from build123d import *

# Parameters (mm, degrees)
CROQUIS1_W                       = 60
CROQUIS1_H                       = 60
SALIENTE_EXTRUIR1_DEPTH          = 73
CORTAR_EXTRUIR1_REACH            = 101.141
CROQUIS2_W                       = 50
CROQUIS2_H                       = 69.5
CORTAR_EXTRUIR2_REACH            = 86.433
CROQUIS3_R                       = 2
CHAFL_N1_SIZE                    = 5
TALADRO_DE_MARGEN_PARA_M31_D     = 3.4
TALADRO_DE_MARGEN_PARA_M31_DEPTH = 40
TALADRO_DE_MARGEN_PARA_M31_TIP   = 1.021463052
TALADRO_DE_MARGEN_PARA_M32_D     = 3.4
TALADRO_DE_MARGEN_PARA_M32_DEPTH = 40
TALADRO_DE_MARGEN_PARA_M32_TIP   = 1.021463052
TALADRO_DE_MARGEN_PARA_M33_D     = 3.4
TALADRO_DE_MARGEN_PARA_M33_DEPTH = 40
TALADRO_DE_MARGEN_PARA_M33_TIP   = 1.021463052
CROQUIS11_W                      = 60
CROQUIS11_H                      = 3.5
SALIENTE_EXTRUIR2_DEPTH          = 40
CHAFL_N2_SIZE                    = 40
CORTAR_EXTRUIR3_REACH            = 107.494
CROQUIS12_R                      = 2.5
CROQUIS14_R                      = 10
SALIENTE_EXTRUIR3_DEPTH          = 7
CROQUIS15_R                      = 10
SALIENTE_EXTRUIR4_DEPTH          = 2
CROQUIS13_R                      = 8
CORTAR_EXTRUIR5_DEPTH            = 5
CROQUIS16_R                      = 5
CORTAR_EXTRUIR6_DEPTH            = 5
CROQUIS17_R                      = 4.5
CORTAR_EXTRUIR7_DEPTH            = 16


with BuildPart() as part:
    # Croquis1 → Saliente-Extruir1 (new body)
    with BuildSketch(Plane(origin=(0, 0, 0), x_dir=(1, 0, 0), z_dir=(0, 1, 0))):
        Rectangle(CROQUIS1_W, CROQUIS1_H)
    extrude(amount=SALIENTE_EXTRUIR1_DEPTH)

    # Croquis2 → Cortar-Extruir1 (cut, up to next)
    with BuildSketch(Plane.XY.offset(30), mode=Mode.PRIVATE) as cortar_extruir1_sk1:
        with Locations((0, 34.75)):
            Rectangle(CROQUIS2_W, CROQUIS2_H)
    cortar_extruir1_tool1 = extrude(cortar_extruir1_sk1.sketch, amount=-CORTAR_EXTRUIR1_REACH, mode=Mode.PRIVATE) & part.part
    add(cortar_extruir1_tool1.solids().sort_by_distance((0, 34.75, 30))[0], mode=Mode.SUBTRACT)

    # Croquis3 → Cortar-Extruir2 (cut, up to next)
    with BuildSketch(Plane(origin=(0, 73, 0), x_dir=(1, 0, 0), z_dir=(0, 1, 0)), mode=Mode.PRIVATE) as cortar_extruir2_sk1:
        with Locations(Location((-8.5, -5.5, 0), (0, 0, 270))):
            Circle(CROQUIS3_R)
    cortar_extruir2_tool1 = extrude(cortar_extruir2_sk1.sketch, amount=-CORTAR_EXTRUIR2_REACH, mode=Mode.PRIVATE) & part.part
    # Croquis3 → Cortar-Extruir2 (cut, up to next)
    with BuildSketch(Plane(origin=(0, 73, 0), x_dir=(1, 0, 0), z_dir=(0, 1, 0)), mode=Mode.PRIVATE) as cortar_extruir2_sk2:
        with Locations(Location((8.5, -5.5, 0), (0, 0, 270))):
            Circle(CROQUIS3_R)
    cortar_extruir2_tool2 = extrude(cortar_extruir2_sk2.sketch, amount=-CORTAR_EXTRUIR2_REACH, mode=Mode.PRIVATE) & part.part
    add(cortar_extruir2_tool1.solids().sort_by_distance((-8.5, 73, 5.5))[0], mode=Mode.SUBTRACT)
    add(cortar_extruir2_tool2.solids().sort_by_distance((8.5, 73, 5.5))[0], mode=Mode.SUBTRACT)

    # Chaflán1
    chafl_n1_edges = [part.edges().sort_by_distance(p)[0] for p in [
        (-25, 69.5, 0),
        (25, 69.5, 0),
    ]]
    chamfer(chafl_n1_edges, length=CHAFL_N1_SIZE)

    # Taladro de margen para M31
    with Locations(Plane.XZ):
        with Locations((27.5, -20), (27.5, 20)):
            Hole(TALADRO_DE_MARGEN_PARA_M31_D / 2, depth=TALADRO_DE_MARGEN_PARA_M31_DEPTH)
            with Locations((0, 0, -(TALADRO_DE_MARGEN_PARA_M31_DEPTH + TALADRO_DE_MARGEN_PARA_M31_TIP / 2))):  # 118° drill point
                Cone(0, TALADRO_DE_MARGEN_PARA_M31_D / 2, TALADRO_DE_MARGEN_PARA_M31_TIP, mode=Mode.SUBTRACT)

    # Taladro de margen para M32
    with Locations(Plane.XZ):
        with Locations((-27.5, 20), (-27.5, -20)):
            Hole(TALADRO_DE_MARGEN_PARA_M32_D / 2, depth=TALADRO_DE_MARGEN_PARA_M32_DEPTH)
            with Locations((0, 0, -(TALADRO_DE_MARGEN_PARA_M32_DEPTH + TALADRO_DE_MARGEN_PARA_M32_TIP / 2))):  # 118° drill point
                Cone(0, TALADRO_DE_MARGEN_PARA_M32_D / 2, TALADRO_DE_MARGEN_PARA_M32_TIP, mode=Mode.SUBTRACT)

    # Taladro de margen para M33
    with Locations(Plane.XZ):
        with Locations((-27.5, 0), (27.5, 1.783505525)):
            Hole(TALADRO_DE_MARGEN_PARA_M33_D / 2, depth=TALADRO_DE_MARGEN_PARA_M33_DEPTH)
            with Locations((0, 0, -(TALADRO_DE_MARGEN_PARA_M33_DEPTH + TALADRO_DE_MARGEN_PARA_M33_TIP / 2))):  # 118° drill point
                Cone(0, TALADRO_DE_MARGEN_PARA_M33_D / 2, TALADRO_DE_MARGEN_PARA_M33_TIP, mode=Mode.SUBTRACT)

    # Croquis11 → Saliente-Extruir2 (add)
    with BuildSketch(Plane.XY.offset(30)):
        with Locations((0, 71.25)):
            Rectangle(CROQUIS11_W, CROQUIS11_H)
    extrude(amount=SALIENTE_EXTRUIR2_DEPTH)

    # Chaflán2
    # the kernel refuses this chamfer: 40 mm, written as the material it adds along each edge
    with BuildSketch(Plane(origin=(30, 69.5, 30), x_dir=(0, -0.9996219169112968, -0.027495876610586403), z_dir=(-1, 0, 0))) as chafl_n2_piece_1_section:
        Polygon((CHAFL_N2_SIZE * 0.999621916911, CHAFL_N2_SIZE * 0.0274958766106), (-CHAFL_N2_SIZE * 0.0274958766106, CHAFL_N2_SIZE * 0.999621916911), (0, 0), align=None)
    chafl_n2_piece_1 = extrude(amount=112.867319519, mode=Mode.PRIVATE)
    chafl_n2_piece_1 = split(chafl_n2_piece_1, bisect_by=Plane(origin=(25, 65.769230769, 48.134615385), z_dir=(1, 0, 0)), keep=Keep.TOP, mode=Mode.PRIVATE)
    add(chafl_n2_piece_1)
    with BuildSketch(Plane(origin=(132.867319519, 69.5, 30), x_dir=(0, -0.9996219169112968, -0.027495876610586403), z_dir=(-1, 0, 0))) as chafl_n2_piece_2_section:
        Polygon((CHAFL_N2_SIZE * 0.999621916911, CHAFL_N2_SIZE * 0.0274958766106), (-CHAFL_N2_SIZE * 0.0274958766106, CHAFL_N2_SIZE * 0.999621916911), (0, 0), align=None)
    chafl_n2_piece_2 = extrude(amount=215.734639037, mode=Mode.PRIVATE)
    chafl_n2_piece_2 = split(chafl_n2_piece_2, bisect_by=Plane(origin=(22.472826087, 67.027173913, 49.184782609), z_dir=(0.7071067811865476, 0.7071067811865476, 0)), keep=Keep.TOP, mode=Mode.PRIVATE)
    chafl_n2_piece_2 = split(chafl_n2_piece_2, bisect_by=Plane(origin=(25, 67.869565217, 49.184782609), z_dir=(-1, 0, 0)), keep=Keep.TOP, mode=Mode.PRIVATE)
    add(chafl_n2_piece_2)
    with BuildSketch(Plane(origin=(132.867319519, 69.5, 30), x_dir=(0, -0.9996219169112968, -0.027495876610586403), z_dir=(-1, 0, 0))) as chafl_n2_piece_3_section:
        Polygon((CHAFL_N2_SIZE * 0.999621916911, CHAFL_N2_SIZE * 0.0274958766106), (-CHAFL_N2_SIZE * 0.0274958766106, CHAFL_N2_SIZE * 0.999621916911), (0, 0), align=None)
    chafl_n2_piece_3 = extrude(amount=215.734639037, mode=Mode.PRIVATE)
    chafl_n2_piece_3 = split(chafl_n2_piece_3, bisect_by=Plane(origin=(-30, 67.869565217, 49.184782609), z_dir=(1, 0, 0)), keep=Keep.TOP, mode=Mode.PRIVATE)
    chafl_n2_piece_3 = split(chafl_n2_piece_3, bisect_by=Plane(origin=(-22.472826087, 67.027173913, 49.184782609), z_dir=(-0.7071067811865476, 0.7071067811865476, 0)), keep=Keep.TOP, mode=Mode.PRIVATE)
    add(chafl_n2_piece_3)
    with BuildSketch(Plane(origin=(132.867319519, 69.5, 30), x_dir=(0, -0.9996219169112968, -0.027495876610586403), z_dir=(-1, 0, 0))) as chafl_n2_piece_4_section:
        Polygon((CHAFL_N2_SIZE * 0.999621916911, CHAFL_N2_SIZE * 0.0274958766106), (-CHAFL_N2_SIZE * 0.0274958766106, CHAFL_N2_SIZE * 0.999621916911), (0, 0), align=None)
    chafl_n2_piece_4 = extrude(amount=215.734639037, mode=Mode.PRIVATE)
    chafl_n2_piece_4 = split(chafl_n2_piece_4, bisect_by=Plane(origin=(-25, 51.251968504, 40.875984252), z_dir=(-1, 0, 0)), keep=Keep.TOP, mode=Mode.PRIVATE)
    chafl_n2_piece_4 = split(chafl_n2_piece_4, bisect_by=Plane(origin=(-30, 51.251968504, 40.875984252), z_dir=(1, 0, 0)), keep=Keep.TOP, mode=Mode.PRIVATE)
    add(chafl_n2_piece_4)
    with BuildSketch(Plane(origin=(82.867319519, 69.5, 30), x_dir=(0, -0.9996219169112968, -0.027495876610586403), z_dir=(-1, 0, 0))) as chafl_n2_piece_5_section:
        Polygon((CHAFL_N2_SIZE * 0.999621916911, CHAFL_N2_SIZE * 0.0274958766106), (-CHAFL_N2_SIZE * 0.0274958766106, CHAFL_N2_SIZE * 0.999621916911), (0, 0), align=None)
    chafl_n2_piece_5 = extrude(amount=215.734639037, mode=Mode.PRIVATE)
    chafl_n2_piece_5 = split(chafl_n2_piece_5, bisect_by=Plane(origin=(30, 65.769230769, 48.134615385), z_dir=(-1, 0, 0)), keep=Keep.TOP, mode=Mode.PRIVATE)
    chafl_n2_piece_5 = split(chafl_n2_piece_5, bisect_by=Plane(origin=(25, 65.769230769, 48.134615385), z_dir=(1, 0, 0)), keep=Keep.TOP, mode=Mode.PRIVATE)
    add(chafl_n2_piece_5)
    with BuildSketch(Plane(origin=(82.867319519, 69.5, 30), x_dir=(0, -0.9996219169112968, -0.027495876610586403), z_dir=(-1, 0, 0))) as chafl_n2_piece_6_section:
        Polygon((CHAFL_N2_SIZE * 0.999621916911, CHAFL_N2_SIZE * 0.0274958766106), (-CHAFL_N2_SIZE * 0.0274958766106, CHAFL_N2_SIZE * 0.999621916911), (0, 0), align=None)
    chafl_n2_piece_6 = extrude(amount=215.734639037, mode=Mode.PRIVATE)
    chafl_n2_piece_6 = split(chafl_n2_piece_6, bisect_by=Plane(origin=(22.472826087, 67.027173913, 49.184782609), z_dir=(0.7071067811865476, 0.7071067811865476, 0)), keep=Keep.TOP, mode=Mode.PRIVATE)
    chafl_n2_piece_6 = split(chafl_n2_piece_6, bisect_by=Plane(origin=(25, 67.869565217, 49.184782609), z_dir=(-1, 0, 0)), keep=Keep.TOP, mode=Mode.PRIVATE)
    add(chafl_n2_piece_6)
    with BuildSketch(Plane(origin=(82.867319519, 69.5, 30), x_dir=(0, -0.9996219169112968, -0.027495876610586403), z_dir=(-1, 0, 0))) as chafl_n2_piece_7_section:
        Polygon((CHAFL_N2_SIZE * 0.999621916911, CHAFL_N2_SIZE * 0.0274958766106), (-CHAFL_N2_SIZE * 0.0274958766106, CHAFL_N2_SIZE * 0.999621916911), (0, 0), align=None)
    chafl_n2_piece_7 = extrude(amount=112.867319519, mode=Mode.PRIVATE)
    chafl_n2_piece_7 = split(chafl_n2_piece_7, bisect_by=Plane(origin=(-22.472826087, 67.027173913, 49.184782609), z_dir=(-0.7071067811865476, 0.7071067811865476, 0)), keep=Keep.TOP, mode=Mode.PRIVATE)
    add(chafl_n2_piece_7)
    with BuildSketch(Plane(origin=(82.867319519, 69.5, 30), x_dir=(0, -0.9996219169112968, -0.027495876610586403), z_dir=(-1, 0, 0))) as chafl_n2_piece_8_section:
        Polygon((CHAFL_N2_SIZE * 0.999621916911, CHAFL_N2_SIZE * 0.0274958766106), (-CHAFL_N2_SIZE * 0.0274958766106, CHAFL_N2_SIZE * 0.999621916911), (0, 0), align=None)
    chafl_n2_piece_8 = extrude(amount=112.867319519, mode=Mode.PRIVATE)
    chafl_n2_piece_8 = split(chafl_n2_piece_8, bisect_by=Plane(origin=(-25, 51.251968504, 40.875984252), z_dir=(-1, 0, 0)), keep=Keep.TOP, mode=Mode.PRIVATE)
    add(chafl_n2_piece_8)

    # Croquis12 → Cortar-Extruir3 (cut, up to next)
    with BuildSketch(Plane(origin=(0, 73, 0), x_dir=(1, 0, 0), z_dir=(0, 1, 0)), mode=Mode.PRIVATE) as cortar_extruir3_sk1:
        with Locations(Location((0, -60, 0), (0, 0, 270))):
            Circle(CROQUIS12_R)
    cortar_extruir3_tool1 = extrude(cortar_extruir3_sk1.sketch, amount=-CORTAR_EXTRUIR3_REACH, mode=Mode.PRIVATE) & part.part
    add(cortar_extruir3_tool1.solids().sort_by_distance((0, 73, 60))[0], mode=Mode.SUBTRACT)

    # Croquis14 → Saliente-Extruir3 (add)
    with BuildSketch(Plane(origin=(0, 73, 0), x_dir=(1, 0, 0), z_dir=(0, 1, 0))):
        with Locations(Location((0, -60, 0), (0, 0, 270))):
            Circle(CROQUIS14_R)
    extrude(amount=-SALIENTE_EXTRUIR3_DEPTH)

    # Croquis15 → Saliente-Extruir4 (add)
    with BuildSketch(Plane.XZ.offset(-66)):
        with Locations(Location((0, 60, 0), (0, 0, 90))):
            Circle(CROQUIS15_R)
    extrude(amount=SALIENTE_EXTRUIR4_DEPTH)

    # Croquis13 → Cortar-Extruir5 (cut)
    with BuildSketch(Plane(origin=(0, 73, 0), x_dir=(1, 0, 0), z_dir=(0, 1, 0))):
        with Locations(Location((0, -60, 0), (0, 0, 270))):
            Circle(CROQUIS13_R)
    extrude(amount=-CORTAR_EXTRUIR5_DEPTH, mode=Mode.SUBTRACT)

    # Croquis16 → Cortar-Extruir6 (cut)
    with BuildSketch(Plane(origin=(0, 68, 0), x_dir=(1, 0, 0), z_dir=(0, 1, 0))):
        with Locations(Location((0, -60, 0), (0, 0, 270))):
            Circle(CROQUIS16_R)
    extrude(amount=-CORTAR_EXTRUIR6_DEPTH, mode=Mode.SUBTRACT)

    # Croquis17 → Cortar-Extruir7 (cut)
    with BuildSketch(Plane(origin=(0, 73, 0), x_dir=(1, 0, 0), z_dir=(0, 1, 0))):
        with Locations(Location((0, -5.5, 0), (0, 0, 270))):
            Circle(CROQUIS17_R)
    extrude(amount=-CORTAR_EXTRUIR7_DEPTH, mode=Mode.SUBTRACT)


solid = part.part
Verification items for the finished model (mm, model axes). A direction names the side the tool comes from. Coordinates: 2 decimals unless noted, no trailing zeros. Order: outer loops, then holes, each group sorted by start corner. A loop starts at its lowest first (then second) coordinate and runs counter-clockwise, first axis right, second up. Notation, with made-up numbers: (89, -35.75) -> (105, -35.75) arc R27 ccw to (105, -7.75) -> close; hole circle Ø5 at (24, 52). An arc over 180 degrees is marked (long way). Put each result on its own line as item: value. Start each with the question number.
1. Cross-section at D-D, the plane x = 3. Record the boundary of the cut face in (y, z).
2. Access from +Z, -Z, +X, -X, +Y, -Y to the whole of each face (thin tool, end or side, straight path). Record for faces 5 (the flat face through (0.1, 68, 65.2)), 6 (the flat face through (2, 64, 55)), 7 (the cylindrical face through (25.93, 20.28, 19.35)), 8 (the cylindrical face through (1.352, 71.274, 9.792)), 9 (the flat face through (27, 15, 30)).
3. Material ranges on L1, parallel to Z at x = 27.5, y = 17; L2, parallel to X at y = 21, z = -20; L3, parallel to X at y = 47, z = 22.5, recorded low to high. Write a range as [from, to].
4. Cross-section at A-A, the plane y = 43. Record the boundary of the cut face in (x, z).
5. Mould release check, pull along X, two halves, no side actions. Record for faces 1 (the flat face through (30, 37, 9)), 2 (the conical face through (-27.564, 40.844, -20.288)), 3 (the cylindrical face through (9.852, 71.274, 4.026)), 4 (the flat face through (-27.2, 49.2, 49.7)): released by +X, released by -X, zero draft, split by the parting line, or undercut.
6. Cross-section at B-B, the plane z = 5.5. Record the boundary of the cut face in (x, y), then the cut area to 4 significant figures.
7. Go/stop test with flat-tipped pins: pin 1 Ø10 at (x, z) = (10, 13) entering from -Y; pin 2 Ø2.5 at (x, z) = (-8.5, 5.5) entering from +Y; pin 3 Ø11.5 at (x, z) = (0, 60) entering from +Y; pin 4 Ø1.5 at (x, y) = (26.5, 10.5) entering from +Z. Record where each tip stops, or that it passes through.
8. Cross-section at C-C, the plane z = 42. Record the boundary of the cut face in (x, y).
Computed:
1. outline: (64, 50.46) -> (69.5, 50.46) -> (69.5, 8.85) -> (73, 8.85) -> (73, 52.58) -> (68, 52.58) -> (68, 56) -> (64, 56) -> close; (64, 64) -> (68, 64) -> (68, 67.42) -> (73, 67.42) -> (73, 70) -> (69.5, 70) -> (69.5, 69.54) -> (64, 69.54) -> close; (69.5, -30) -> (73, -30) -> (73, 2.15) -> (69.5, 2.15) -> close
2. face 5: +Y
2. face 6: +Z, -Z, -Y
2. face 7: -Y
2. face 8: +Y, -Y
2. face 9: +Z, +X, -X, -Y
3. L1: [-30, -21.7], [-18.3, 0.08], [3.48, 18.3], [21.7, 30]
3. L2: [-30, -29.2], [-25.8, -25], [25, 25.8], [29.2, 30]
3. L3: [-30, -25], [25, 30]
4. outline: (-30, -30) -> (-25, -30) -> (-25, 43.5) -> (-30, 43.5) -> close; (25, -30) -> (30, -30) -> (30, 43.5) -> (25, 43.5) -> close
5. face 1: released by +X
5. face 2: undercut
5. face 3: undercut
5. face 4: zero draft
6. outline: (-30, 0) -> (-25, 0) -> (-25, 64.5) -> (-20, 69.5) -> (-10.5, 69.5) -> (-10.5, 73) -> (-30, 73) -> close; (-6.5, 69.5) -> (-4.5, 69.5) -> (-4.5, 73) -> (-6.5, 73) -> close; (4.5, 69.5) -> (6.5, 69.5) -> (6.5, 73) -> (4.5, 73) -> close; (10.5, 69.5) -> (20, 69.5) -> (25, 64.5) -> (25, 0) -> (30, 0) -> (30, 73) -> (10.5, 73) -> close
6. area: 870.5 mm2
7. pin 1: y = 69.5
7. pin 2: through
7. pin 3: y = 68
7. pin 4: z = 30
8. outline: (-30, 41.5) -> (-25, 41.5) -> (-25, 64.5) -> (-20, 69.5) -> (20, 69.5) -> (25, 64.5) -> (25, 41.5) -> (30, 41.5) -> (30, 73) -> (-30, 73) -> close
